Verification items for this drawing (mm, ordinates from the low corner). A direction names the side the tool comes from. Coordinates: 2 decimals unless noted, no trailing zeros. Order: outer loops, then holes, each group sorted by start corner. A loop starts at its lowest first (then second) coordinate and runs counter-clockwise, first axis right, second up. Notation, with made-up numbers: M 56,-6.5 L 99,-6.5 A13 ccw 99,14.5 Z; hole C 73,23.5 d5. An arc over 180 degrees is marked long. One line per item, written item: value. Start each with the question number.
1) Go/stop test with flat-tipped pins: P1, Ø4, axis at x = 22, y = 18, coming from the -Z side; P2, Ø1.5, axis at y = 12, z = 13, coming from the -X side; P3, Ø2, axis at x = 8.5, y = 9, coming from the +Z side; P4, Ø10, axis at x = 12.5, z = 19, coming from the +Y side. Record where each tip stops, or that it passes through.
2) Access from +Z, -Z, +X, -X, +Y, -Y to the whole of each face (thin tool, end or side, straight path). Record for the marked faces 1 and 2.
3) Draft check along Y on the marked faces 3, 4 and 5. Enter one of: pulls with the +Y half, pulls with the -Y half, needs draft (parallel to the pull), parting line crosses it, or undercut.
4) Sectioned sample at A-A, the plane x = 2.5. Enter the section's corners in (y, z).
5) Sectioned sample at B-B, the plane x = 13.5. Enter the section's corners in (y, z), then the cut area to 3 significant figures.
6) Thickness scan on L1, parallel to X at y = 12.35, z = 12.5; L2, parallel to Y at x = 21, z = 12.5; L3, parallel to X at y = 15.75, z = 10.5. Record the ranges inside material, lowest first. Write a range as from..to.
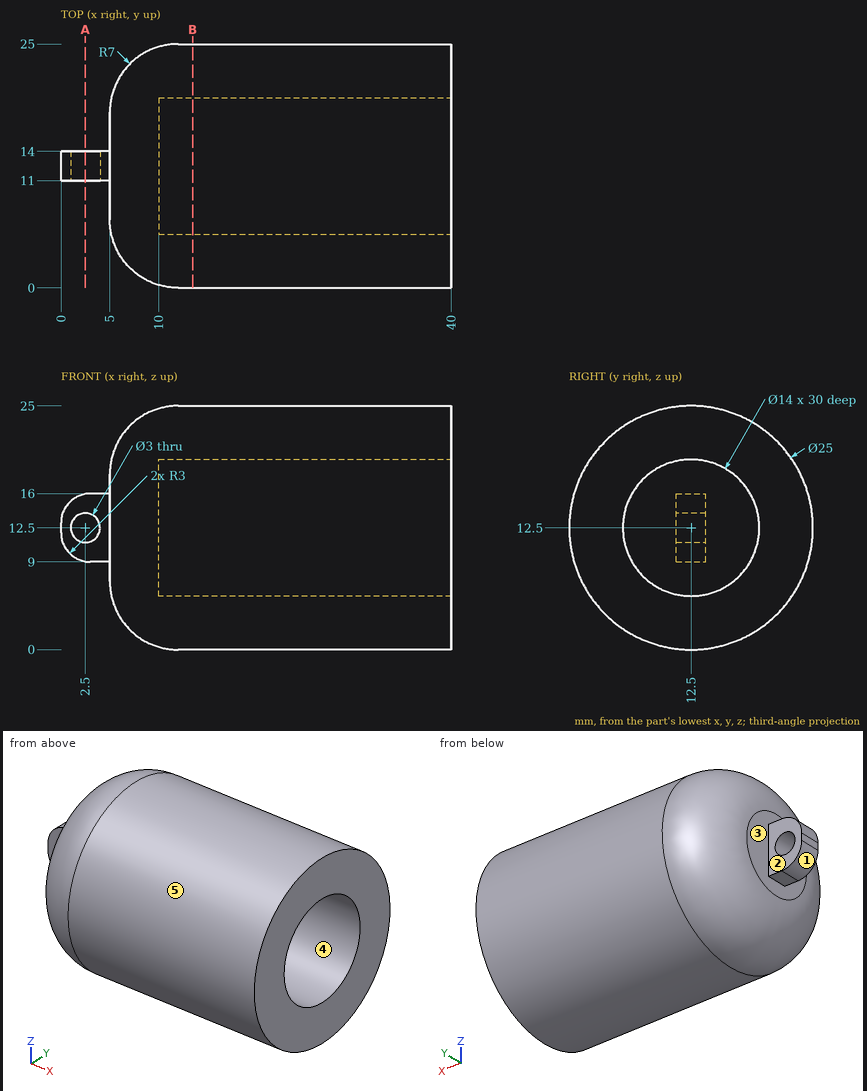
Final values:
1. P1: stops at z = 0.5
1. P2: stops at x = 0
1. P3: stops at z = 24.1
1. P4: stops at y = 24.91
2. face 1: -Z, -X, +Y, -Y
2. face 2: +Z, -Z, -X, +Y
3. face 3: needs draft
3. face 4: undercut
3. face 5: parting line crosses it
4. outline: M 11,9.04 L 14,9.04 L 14,11 L 11,11 Z; M 11,14 L 14,14 L 14,15.96 L 11,15.96 Z
5. outline: C 12.5,12.5 d25; hole C 12.5,12.5 d14
5. area: 337 mm^2
6. L1: x = 0..1, 4..10
6. L2: y = 0..5.5, 19.5..25
6. L3: x = 5..10
